Source: CAD feature listing. Evaluate the final solid. Frame: model axes, mm. Coordinates: 2 decimals unless noted, no trailing zeros. Order: outer loops, then holes, each group sorted by start corner. A loop starts at its lowest first (then second) coordinate and runs counter-clockwise, first axis right, second up. Notation, with made-up numbers: (29, 65.5) -> (82, 65.5) arc R20 ccw to (82, 82.5) -> close; hole circle Ø2 at (0.5, -12). An arc over 180 degrees is marked (long way). Write item = value, one per line. Start each with the question number.
Item 1: Section query D-D (y = 22.75). Output: boundary loops of the cut face in (x, z).
Item 2: Contact query for flat-ended pins moving along their axis: pin 1 (1.5 mm diameter, centred on x = 172, y = 20.5, fed in from +Z); pin 2 (1 mm diameter, centred on y = 16, z = -2, fed in from -X). Output: stop coordinate, or through.
Item 3: Section query B-B (x = 187.3). Output: boundary loops of the cut face in (y, z) (3 decimals), then the cut area to 3 significant figures.
Item 4: Ray query, line 1 along Y through (x, z) = (187.3, -4) (3 decimals); line 2 along X through (y, z) = (18.5, -4.75) (1 decimal); line 3 along X through (y, z) = (4.25, -2.5). Return the intervals inside material, ascending. Write a range as [from, to].
Item 5: Section query A-A (y = 12.7). Output: boundary loops of the cut face in (x, z) (3 decimals).
Item 6: Section query C-C (z = -5.25). Output: boundary loops of the cut face in (x, y) (3 decimals), then the cut area to 3 significant figures.
Item 7: Mould query, pull axis X, two halves, no side actions, for faces 1 (the flat face through (106, 0, -3)), 2 (the cylindrical face through (1.386, 12.584, -3.131)), 3 (the cylindrical face through (6.805, 10.768, -3.131)). Classes: released by +X, released by -X, zero draft, split by the parting line, or undercut.
```python
from build123d import *

# Parameters (mm, degrees)
SKETCH1_W           = 6.35
SKETCH1_H           = 25.4
BOSS_EXTRUDE1_DEPTH = 200
SKETCH2_R           = 3.175
CUT_EXTRUDE1_DEPTH  = 202.706426521
SKETCH3_R           = 3.175
CUT_EXTRUDE2_DEPTH  = 202.706426521
SKETCH6_R           = 1.5
CUT_EXTRUDE3_DEPTH  = 202.706426521


with BuildPart() as part:
    # Sketch1 → Boss-Extrude1 (new body)
    with BuildSketch(Plane(origin=(0, 0, 0), x_dir=(0, 0, -1), z_dir=(1, 0, 0))):
        with Locations((3.175, 12.7)):
            Rectangle(SKETCH1_W, SKETCH1_H)
    extrude(amount=BOSS_EXTRUDE1_DEPTH)

    # Sketch2 → Cut-Extrude1 (cut, through all)
    with BuildSketch(Plane.XY):
        with Locations((187.3, 12.7)):
            Circle(SKETCH2_R)
    extrude(amount=-CUT_EXTRUDE1_DEPTH, mode=Mode.SUBTRACT)

    # Sketch3 → Cut-Extrude2 (cut, through all)
    with BuildSketch(Plane.XY):
        with Locations((9.325, 12.7)):
            Circle(SKETCH3_R)
        with BuildLine():
            Line((15.442045256, 25.4), (-1, 25.4))
            Line((-1, 25.4), (-1, 0))
            Line((-1, 0), (15.442045256, 0))
            Line((15.442045256, 0), (5.354999675, 5.823758482))
            ThreePointArc((5.354999675, 5.823758482), (1.385, 12.7), (5.354999675, 19.576241518))
            Line((5.354999675, 19.576241518), (15.442045256, 25.4))
        make_face()
    extrude(amount=-CUT_EXTRUDE2_DEPTH, mode=Mode.SUBTRACT)

    # Sketch6 → Cut-Extrude3 (cut, through all)
    with BuildSketch(Plane.XY):
        with Locations((21.385, 19.4)):
            Circle(SKETCH6_R)
        with Locations((36.385, 19.4)):
            Circle(SKETCH6_R)
    extrude(amount=-CUT_EXTRUDE3_DEPTH, mode=Mode.SUBTRACT)


solid = part.part
```
Computed:
q1.outline = (10.85, -6.35) -> (200, -6.35) -> (200, 0) -> (10.85, 0) -> close
q2.pin_1 = 0
q2.pin_2 = 1.9
q3.outline = (0, -6.35) -> (9.525, -6.35) -> (9.525, 0) -> (0, 0) -> close; (15.875, -6.35) -> (25.4, -6.35) -> (25.4, 0) -> (15.875, 0) -> close
q3.area = 121 mm^2
q4.line_1 = [0, 9.525], [15.875, 25.4]
q4.line_2 = [3.9, 20.2], [22.6, 35.2], [37.6, 200]
q4.line_3 = [8.08, 200]
q5.outline = (1.385, -6.35) -> (6.15, -6.35) -> (6.15, 0) -> (1.385, 0) -> close; (12.5, -6.35) -> (184.125, -6.35) -> (184.125, 0) -> (12.5, 0) -> close; (190.475, -6.35) -> (200, -6.35) -> (200, 0) -> (190.475, 0) -> close
q6.outline = (5.355, 5.824) -> (15.442, 0) -> (200, 0) -> (200, 25.4) -> (15.442, 25.4) -> (5.355, 19.576) arc R7.94 ccw to start; hole circle Ø6.35 at (9.325, 12.7); hole circle Ø3 at (21.385, 19.4); hole circle Ø3 at (36.385, 19.4); hole circle Ø6.35 at (187.3, 12.7)
q6.area = 4,850 mm^2
q7.face_1 = zero draft
q7.face_2 = released by -X
q7.face_3 = undercut
